The model under review builds one solid part; all positions refer to its coordinate system, in mm. A direction names the side the tool comes from. Coordinates: 2 decimals unless noted, no trailing zeros. Order: outer loops, then holes, each group sorted by start corner. A loop starts at its lowest first (then second) coordinate and runs counter-clockwise, first axis right, second up. Notation, with made-up numbers: M 35.25,50.5 L 55.25,50.5 A9 ccw 55.25,57.5 Z; hole C 49,9.5 d1. An arc over 180 degrees is marked long. Write each question's results on one line, items separated by ' | '.
from build123d import *

# Parameters (mm, degrees)
F0_W     = 8
F0_H     = 8
F1_DEPTH = 120
F2_W     = 8
F2_H     = 8
F3_DEPTH = 8
F4_W     = 8
F4_H     = 8
F5_DEPTH = 4
F6_W     = 17
F6_H     = 8
F6_W_2   = 8
F7_DEPTH = 10
F8_R     = 3.99999


# Not quite as in the source:
# - a fillet or chamfer is up to 0.001 mm smaller than in the source, because OpenCascade refuses the exact size


with BuildPart() as f1:
    # F0 (on Right) → F1 (new body)
    with BuildSketch(Plane.YZ):
        Rectangle(F0_W, F0_H)
    extrude(amount=F1_DEPTH)

    # F2 (on face) → F3 (join)
    with BuildSketch(Plane.XY.offset(4)):
        with Locations((4, 0)):
            Rectangle(F2_W, F2_H)
    extrude(amount=F3_DEPTH)

    # F4 (on face) → F5 (join)
    with BuildSketch(Plane(origin=(0, 0, -4), x_dir=(1, 0, 0), z_dir=(0, 0, -1))):
        with Locations((116, 0)):
            Rectangle(F4_W, F4_H)
    extrude(amount=F5_DEPTH)

    # F6 (on face) → F7 (join)
    with BuildSketch(Plane(origin=(0, 0, -8), x_dir=(1, 0, 0), z_dir=(0, 0, -1))):
        with Locations((103.5, 0)):
            Rectangle(F6_W, F6_H)
        with Locations((116, 0)):
            Rectangle(F6_W_2, F6_H)
    extrude(amount=F7_DEPTH)

    # F8 (radius 4 in the source; OpenCascade refuses exactly that, so slightly less here)
    f8_edges = [f1.edges().sort_by_distance(p)[0] for p in [
        (95, -4, -13),
        (95, 4, -13),
    ]]
    fillet(f8_edges, radius=F8_R)


solid = f1.part
1) For pin 1 (1 mm diameter, centred on x = 36.5, y = 0, fed in from +Z); pin 2 (4 mm diameter, centred on x = 43, y = -1.5, fed in from -Z); pin 3 (4 mm diameter, centred on y = -1, z = 7, fed in from +X); pin 4 (5 mm diameter, centred on x = 84.5, z = -8.5, fed in from +Y), all flat-tipped, find the tip position at first contact; note any pin that passes through.
Solutions:
pin 1: z = 4 | pin 2: z = -4 | pin 3: x = 8 | pin 4: through
2) For faces 4 (the flat face through (8, 0, 8)), 5 (the flat face through (103, 0, -8)), 6 (the cylindrical face through (96.141, -2.797, -13.07)), list the 3-axis set-ups (+Z, -Z, +X, -X, +Y, -Y) from which the entire face can be reached by the end or side of a thin tool; tool diameter is ignored.
Solutions:
face 4: +Z, +X, +Y, -Y | face 5: -X, +Y, -Y | face 6: -Z, -X, -Y
3) Take a section at A-A on x = 109.5. State the section outline as (y, z) points.
Solutions:
outline: M -4,-18 L 4,-18 L 4,-8 L -4,-8 Z; M -4,-4 L 4,-4 L 4,4 L -4,4 Z
4) The part is to be moulded in two halves that separate along Z. For faces 1 (the flat face through (107, 0, -18)), 2 (the flat face through (112, 0, -6)), 3 (the flat face through (120, 0, -7)), say which applies: pulls with the +Z half, pulls with the -Z half, needs draft (parallel to the pull), parting line crosses it, or undercut.
Solutions:
face 1: pulls with the -Z half | face 2: undercut | face 3: needs draft
5) To check wall thickness, follow line 1 along Z through (x, y) = (95.5, 0.25); line 2 along X through (y, z) = (3, -4.25); line 3 along Z through (x, y) = (82, 3). State the ranges of each line that lie inside material, in increasing order.
Solutions:
line 1: -18 to -8, -4 to 4 | line 2: 112 to 120 | line 3: -4 to 4
6) Take a section at D-D on x = 20.5. State the section outline as (y, z) points, plus the area to 3 significant figures.
Solutions:
outline: M -4,-4 L 4,-4 L 4,4 L -4,4 Z | area: 64.0 mm2
7) Take a section at B-B on y = 1. State the section outline as (x, z) points.
Solutions:
outline: M 0,-4 L 112,-4 L 112,-8 L 95.13,-8 L 95.13,-18 L 120,-18 L 120,4 L 8,4 L 8,12 L 0,12 Z
